Geometry check sheet. Reference: the model listing, model coordinates, mm. Face numbers are marked on the shaded views. A direction names the side the tool comes from. Coordinates: 2 decimals unless noted, no trailing zeros. Loops run counter-clockwise (first coordinate to the right, second up) from the corner with the lowest first, then second, coordinate; pieces in that order, holes last.
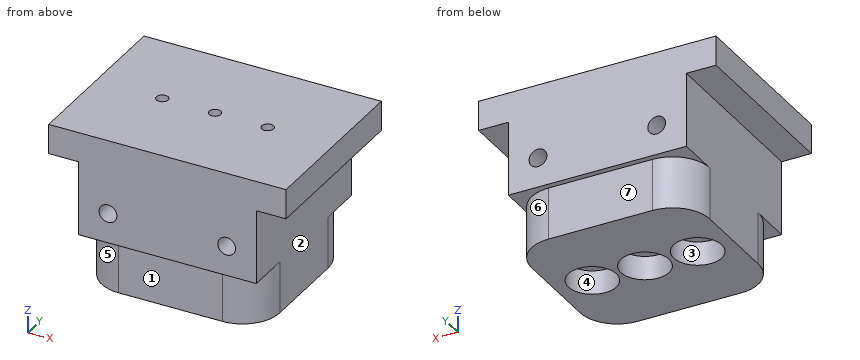
from build123d import *

# Parameters (mm, degrees)
BOSS_EXTRUDE1_DEPTH     = 11.8
BOSS_EXTRUDE2_DEPTH     = 10.5
CUT_EXTRUDE1_DEPTH      = 18.705648816
CUT_EXTRUDE1_DEPTH_BACK = 18.705648816
SKETCH2_R               = 0.6
SKETCH5_R               = 1.625
CUT_EXTRUDE2_DEPTH      = 1.6
CUT_EXTRUDE5_DEPTH      = 17.806248838
CUT_EXTRUDE5_DEPTH_BACK = 17.806248838
SKETCH7_R               = 0.4


with BuildPart() as part:
    # Sketch1 → Boss-Extrude1 (new body)
    with BuildSketch(Plane(origin=(0, 0, 0), x_dir=(1, 0, 0), z_dir=(0, 1, 0))):
        Polygon((0, 0), (8, 0), (8, 2), (6, 2), (6, 7), (-6, 7), (-6, 2), (-8, 2), (-8, 0), align=None)
    extrude(amount=BOSS_EXTRUDE1_DEPTH)

    # Sketch4 → Boss-Extrude2 (add)
    with BuildSketch(Plane.XY):
        with BuildLine():
            Line((-6, 8.9), (-6, 2.9))
            ThreePointArc((-6, 2.9), (-5.267766953, 1.132233047), (-3.5, 0.4))
            Line((-3.5, 0.4), (3.5, 0.4))
            ThreePointArc((3.5, 0.4), (5.267766953, 1.132233047), (6, 2.9))
            Line((6, 2.9), (6, 8.9))
            ThreePointArc((6, 8.9), (5.267766953, 10.667766953), (3.5, 11.4))
            Line((3.5, 11.4), (-3.5, 11.4))
            ThreePointArc((-3.5, 11.4), (-5.267766953, 10.667766953), (-6, 8.9))
        make_face()
    extrude(amount=-BOSS_EXTRUDE2_DEPTH)

    # Sketch2 → Cut-Extrude1 (cut, two sides: drawn at the far end of the back side and taken through both)
    with BuildSketch(Plane(origin=(0, 11.8, 0), x_dir=(1, 0, 0), z_dir=(0, 1, 0)).offset(-CUT_EXTRUDE1_DEPTH_BACK)):
        with Locations(Location((-4, 5, 0), (0, 0, 270))):
            Circle(SKETCH2_R)
        with Locations(Location((4, 5, 0), (0, 0, 270))):
            Circle(SKETCH2_R)
    extrude(amount=CUT_EXTRUDE1_DEPTH + CUT_EXTRUDE1_DEPTH_BACK, mode=Mode.SUBTRACT)

    # Sketch5 → Cut-Extrude2 (cut)
    with BuildSketch(Plane(origin=(0, 0, -10.5), x_dir=(-1, 0, 0), z_dir=(0, 0, -1))):
        with Locations((3.55, 5.9)):
            Circle(SKETCH5_R)
        with Locations((-3.55, 5.9)):
            Circle(SKETCH5_R)
        with Locations((0, 5.9)):
            Circle(SKETCH5_R)
    extrude(amount=-CUT_EXTRUDE2_DEPTH, mode=Mode.SUBTRACT)

    # Sketch7 → Cut-Extrude5 (cut, two sides: drawn at the far end of the back side and taken through both)
    with BuildSketch(Plane(origin=(0, 0, -8.9), x_dir=(-1, 0, 0), z_dir=(0, 0, -1)).offset(-CUT_EXTRUDE5_DEPTH_BACK)):
        with Locations((-3.55, 5.9)):
            Circle(SKETCH7_R)
        with Locations((3.55, 5.9)):
            Circle(SKETCH7_R)
        with Locations((0, 5.9)):
            Circle(SKETCH7_R)
    extrude(amount=CUT_EXTRUDE5_DEPTH + CUT_EXTRUDE5_DEPTH_BACK, mode=Mode.SUBTRACT)


solid = part.part
(1) Sectioned sample at D-D on y = 5.9. State how many separate pieces and enclosed holes the cut face has, and give its area (3 significant figures).
Findings:
separate pieces: 4
enclosed holes: 0
area: 95.8 mm2
(2) Sectioned sample at C-C on x = 7. Record the cut outline in (y, z).
Findings:
outline: (0, -2) - (11.8, -2) - (11.8, 0) - (0, 0) - close
(3) Draft check along Y on the marked faces 1, 2, 3 and 4. Enter one of: +Y half, -Y half, draft (parallel to the pull), parting line (faces both ways), or undercut.
Findings:
face 1: -Y half
face 2: draft
face 3: undercut
face 4: undercut
(4) Scan lines: L1, parallel to Y at x = 0, z = -10.1 (3 decimals); L2, parallel to Y at x = -3.55, z = -2.5; L3, parallel to X at y = 3.5, z = -8.5. Record each from-to range of solid material in increasing order.
Findings:
L1: y = 0.4 to 4.275, 7.525 to 11.4
L2: y = 0 to 5.5, 6.3 to 11.8
L3: x = -6 to 6
(5) Gauge pin test, flat ends, axial feed: pin 1 Ø5 at (x, y) = (0, 5.9) entering from +Z; pin 2 Ø1 at (x, y) = (-7.5, 6.5) entering from -Z; pin 3 Ø1.6 at (x, y) = (3.5, 5.5) entering from -Z; pin 4 Ø1 at (y, z) = (8.5, -5) entering from -X. Record the tip position at first contact, or that the pin passes through.
Findings:
pin 1: stops at z = 0
pin 2: stops at z = -2
pin 3: stops at z = -8.9
pin 4: stops at x = -6
(6) Sectioned sample at A-A on z = -2.75. Record the cut outline in (x, y).
Findings:
outline: (-6, 0) - (6, 0) - (6, 11.8) - (-6, 11.8) - close; hole circle Ø0.8 at (-3.55, 5.9); hole circle Ø0.8 at (0, 5.9); hole circle Ø0.8 at (3.55, 5.9)
(7) Access from +Z, -Z, +X, -X, +Y, -Y to the whole of each face (thin tool, end or side, straight path). Record for the marked faces 5, 6 and 7.
Findings:
face 5: -Z, -X, -Y
face 6: -Z, +X, +Y
face 7: -Z, +X, -X, +Y
(8) Sectioned sample at B-B on y = 8.5. Record the cut outline in (x, z).
Findings:
outline: (-8, -2) - (-6, -2) - (-6, -10.5) - (6, -10.5) - (6, -2) - (8, -2) - (8, 0) - (-8, 0) - close; hole circle Ø1.2 at (-4, -5); hole circle Ø1.2 at (4, -5)
